Source: CAD feature listing. Evaluate the final solid. Frame: model axes, mm. Face numbers are marked on the shaded views. A direction names the side the tool comes from. Give positions to 0.01 mm unless a question says otherwise; leave off trailing zeros. Loops run counter-clockwise (first coordinate to the right, second up) from the corner with the lowest first, then second, coordinate; pieces in that order, holes last. Notation, with made-up numbers: (82, 1.5) - (118, 1.5) arc R17 cw to (118, 25.5) - close; hole circle Ø7 at (-28.5, -8). An arc over 180 degrees is marked (long way). Write each question's results on one line, items separated by ' | '. Start each with the question number.
(1) Cut plane A-A on y = 3. Return the cut outline in (x, z).
(2) Cut plane C-C on z = 0. Return the cut outline in (x, y).
(3) Cut plane D-D on y = 0. Return the cut outline in (x, z).
(4) Cut plane B-B on x = -7.75. Return the cut outline in (y, z), then the cut area to 3 significant figures.
(5) Reachability of the marked faces 1, 2, 3, 4 and 5 from +Z, -Z, +X, -X, +Y, -Y: full face, straight path, thin tool, end or side. Return the list, or none.
(6) Pull-direction query (X, two-part tool) for the marked faces 6, 7, 8 and 9; classes: pulls with the +X half, pulls with the -X half, needs draft (parallel to the pull), parting line crosses it, or undercut.
(7) Material intervals for line 1 along X through (y, z) = (3, -0.1); line 2 along Y through (x, z) = (-0.9, 0); line 3 along Y through (x, z) = (-11, 0.8), sorted ascending. Write a range as [from, to].
(8) Contact query for flat-ended pins moving along their axis: pin 1 (1.5 mm diameter, centred on y = -0.5, z = 0.5, fed in from +X); pin 2 (0.6 mm diameter, centred on y = -2.5, z = 0, fed in from -X); pin 3 (1.5 mm diameter, centred on y = 0, z = 0, fed in from +X); pin 4 (2 mm diameter, centred on x = -12.5, z = -0.5, fed in from +Y). Output: stop coordinate, or through.
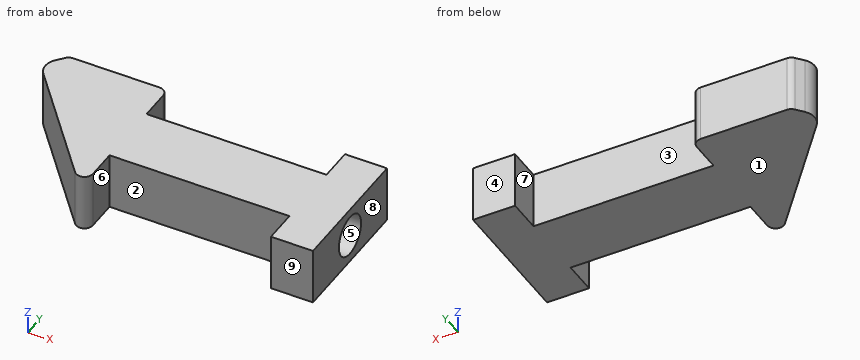
from build123d import *

# Parameters (mm, degrees)
BOSS_EXTRUDE3_DEPTH = 1.7
SKETCH3_R           = 0.95
CUT_EXTRUDE1_DEPTH  = 9.5
SKETCH4_R           = 1.2
CUT_EXTRUDE2_DEPTH  = 2.8


with BuildPart() as part:
    # Sketch2 → Boss-Extrude3 (new body, symmetric)
    with BuildSketch(Plane.XY):
        with BuildLine():
            Line((-18.828250092, 4.3), (-13.7, 4.3))
            ThreePointArc((-13.7, 4.3), (-13.346446609, 4.153553391), (-13.2, 3.8))
            Line((-13.2, 3.8), (-13.2, 2))
            Line((-13.2, 2), (-2.5, 2))
            Line((-2.5, 2), (-2.5, 4))
            Line((-2.5, 4), (0, 4))
            Line((0, 4), (0, -4))
            Line((0, -4), (-2.5, -4))
            Line((-2.5, -4), (-2.5, -2))
            Line((-2.5, -2), (-13.2, -2))
            Line((-13.2, -2), (-13.2, -3.8))
            ThreePointArc((-13.2, -3.8), (-13.528989928, -4.26984631), (-14.083022222, -4.121393805))
            Line((-14.083022222, -4.121393805), (-19.566044443, 2.413017626))
            ThreePointArc((-19.566044443, 2.413017626), (-19.8, 3.055805236), (-19.566044443, 3.698592845))
            Line((-19.566044443, 3.698592845), (-19.211272314, 4.121393805))
            ThreePointArc((-19.211272314, 4.121393805), (-19.039559223, 4.253153894), (-18.828250092, 4.3))
        make_face()
    extrude(amount=BOSS_EXTRUDE3_DEPTH, both=True)

    # Sketch3 → Cut-Extrude1 (cut)
    with BuildSketch(Plane(origin=(0, 0, 0), x_dir=(0, 0, -1), z_dir=(1, 0, 0))):
        Circle(SKETCH3_R)
    extrude(amount=-CUT_EXTRUDE1_DEPTH, mode=Mode.SUBTRACT)

    # Sketch4 → Cut-Extrude2 (cut)
    with BuildSketch(Plane(origin=(0, 0, 0), x_dir=(0, 0, -1), z_dir=(1, 0, 0))):
        Circle(SKETCH4_R)
    extrude(amount=-CUT_EXTRUDE2_DEPTH, mode=Mode.SUBTRACT)


solid = part.part
Ans:
1) outline: (-19.8, -1.7) - (-13.2, -1.7) - (-13.2, 1.7) - (-19.8, 1.7) - close; (-2.5, -1.7) - (0, -1.7) - (0, 1.7) - (-2.5, 1.7) - close
2) outline: (-19.57, 2.41) - (-14.08, -4.12) arc R0.5 ccw to (-13.2, -3.8) - (-13.2, -2) - (-2.5, -2) - (-2.5, -4) - (0, -4) - (0, -1.2) - (-2.8, -1.2) - (-2.8, -0.95) - (-9.5, -0.95) - (-9.5, 0.95) - (-2.8, 0.95) - (-2.8, 1.2) - (0, 1.2) - (0, 4) - (-2.5, 4) - (-2.5, 2) - (-13.2, 2) - (-13.2, 3.8) arc R0.5 ccw to (-13.7, 4.3) - (-18.83, 4.3) arc R0.5 ccw to (-19.21, 4.12) - (-19.57, 3.7) arc R1 ccw to start
3) outline: (-17.54, -1.7) - (0, -1.7) - (0, -1.2) - (-2.8, -1.2) - (-2.8, -0.95) - (-9.5, -0.95) - (-9.5, 0.95) - (-2.8, 0.95) - (-2.8, 1.2) - (0, 1.2) - (0, 1.7) - (-17.54, 1.7) - close
4) outline: (-2, -1.7) - (2, -1.7) - (2, 1.7) - (-2, 1.7) - close; hole circle Ø1.9 at (0, 0) | area: 10.8 mm^2
5) face 1: -Z, +X, -X, +Y, -Y | face 2: +Z, -Z, -Y | face 3: +Z, -Z, +Y | face 4: +Z, -Z, +X, +Y | face 5: +X
6) face 6: undercut | face 7: undercut | face 8: pulls with the +X half | face 9: needs draft
7) line 1: [-19.8, -13.2], [-2.5, 0] | line 2: [-4, -1.2], [1.2, 4] | line 3: [-2, 2]
8) pin 1: x = 0 | pin 2: x = -15.7 | pin 3: x = -9.5 | pin 4: y = 4.26
